The model under review builds one solid part; all positions refer to its coordinate system, in mm. Face numbers are marked on the shaded views. A direction names the side the tool comes from. Round coordinates to 2 decimals unless told otherwise and drop trailing zeros. Order: outer loops, then holes, each group sorted by start corner. A loop starts at its lowest first (then second) coordinate and runs counter-clockwise, first axis right, second up. Notation, with made-up numbers: (-33.75, 67) -> (-14.75, 67) arc R12 ccw to (-14.75, 83) -> close; hole circle Ø3 at (75, 85.5). An arc over 180 degrees is marked (long way). Use a Markdown table: item, result. Add a question column.
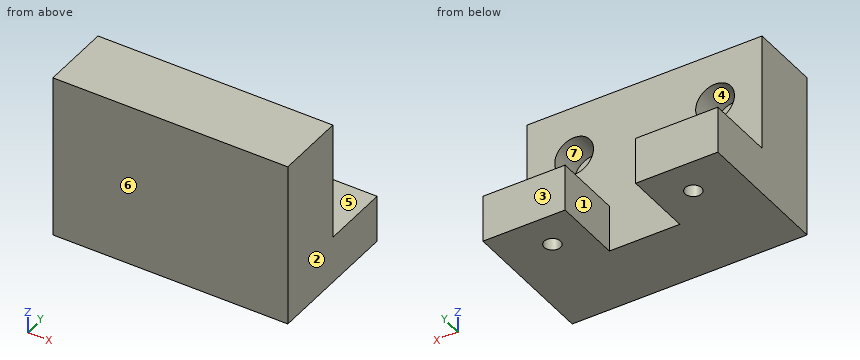
```python
from build123d import *

# Parameters (mm, degrees)
F1_DEPTH = 100
F2_R     = 8.25
F3_DEPTH = 12.954
F4_R     = 3.5
F5_DEPTH = 20
F6_W     = 30
F6_H     = 29.45
F7_DEPTH = 20


with BuildPart() as f1:
    # F0 (on Right) → F1 (new body)
    with BuildSketch(Plane.YZ):
        Polygon((0, 0), (59.45, 0), (59.45, 20), (30, 20), (30, 70), (0, 70), align=None)
    extrude(amount=F1_DEPTH)

    # F2 (on face) → F3 (cut)
    with BuildSketch(Plane(origin=(0, 30, 0), x_dir=(-1, 0, 0), z_dir=(0, 1, 0))):
        with Locations((-80, 48.25)):
            Circle(F2_R)
        with Locations((-20, 48.25)):
            Circle(F2_R)
    extrude(amount=-F3_DEPTH, mode=Mode.SUBTRACT)

    # F4 (on face) → F5 (cut, through all)
    with BuildSketch(Plane.XY.offset(20)):
        with Locations((80, 44.45)):
            Circle(F4_R)
        with Locations((20, 44.45)):
            Circle(F4_R)
    extrude(amount=-F5_DEPTH, mode=Mode.SUBTRACT)

    # F6 (on face) → F7 (cut, through all)
    with BuildSketch(Plane.XY.offset(20)):
        with Locations((50, 44.725)):
            Rectangle(F6_W, F6_H)
    extrude(amount=-F7_DEPTH, mode=Mode.SUBTRACT)


solid = f1.part
```
Q1. For pin 1 (14.5 mm diameter, centred on x = 19, y = 39, fed in from +Z); pin 2 (18 mm diameter, centred on x = 16, z = 47, fed in from +Y); pin 3 (5.5 mm diameter, centred on x = 20, y = 44.45, fed in from -Z), all flat-tipped, find the tip position at first contact; note any pin that passes through.
Q2. Add section A-A, the plane y = 44.45. Give the boundary of the cut face in (x, z), then the cut area to 3 significant figures.
Q3. Draft analysis for pull direction X (two halves, no side actions). For the marked faces 1, 2, 3 and 4, state which applies: released by +X, released by -X, zero draft, split by the parting line, or undercut.
Q4. Add section C-C, the plane y = 32. Give the boundary of the cut face in (x, z), then the cut area to 3 significant figures.
Q5. Add section D-D, the plane z = 48.25. Give the boundary of the cut face in (x, y).
Q6. To check wall thickness, follow line 1 along X through (y, z) = (24, 48); line 2 along Y through (x, z) = (20, 8.75); line 3 along X through (y, z) = (48, 18.5). State the ranges of each line that lie inside material, in increasing order.
Q7. Add section B-B, the plane x = 80. Give the boundary of the cut face in (y, z).
Q8. For the marked faces 5, 6 and 7, list the 3-axis set-ups (+Z, -Z, +X, -X, +Y, -Y) from which the entire face can be reached by the end or side of a thin tool; tool diameter is ignored.
Return value:
| question | item | result |
|---|---|---|
| 1 | pin 1 | z = 20 |
| 1 | pin 2 | y = 30 |
| 1 | pin 3 | through |
| 2 | outline | (0, 0) -> (16.5, 0) -> (16.5, 20) -> (0, 20) -> close; (23.5, 0) -> (35, 0) -> (35, 20) -> (23.5, 20) -> close; (65, 0) -> (76.5, 0) -> (76.5, 20) -> (65, 20) -> close; (83.5, 0) -> (100, 0) -> (100, 20) -> (83.5, 20) -> close |
| 2 | area | 1,120 mm² |
| 3 | face 1 | undercut |
| 3 | face 2 | released by +X |
| 3 | face 3 | zero draft |
| 3 | face 4 | undercut |
| 4 | outline | (0, 0) -> (35, 0) -> (35, 20) -> (0, 20) -> close; (65, 0) -> (100, 0) -> (100, 20) -> (65, 20) -> close |
| 4 | area | 1,400 mm² |
| 5 | outline | (0, 0) -> (100, 0) -> (100, 30) -> (88.25, 30) -> (88.25, 17.05) -> (71.75, 17.05) -> (71.75, 30) -> (28.25, 30) -> (28.25, 17.05) -> (11.75, 17.05) -> (11.75, 30) -> (0, 30) -> close |
| 6 | line 1 | 0 to 11.75, 28.25 to 71.75, 88.25 to 100 |
| 6 | line 2 | 0 to 40.95, 47.95 to 59.45 |
| 6 | line 3 | 0 to 35, 65 to 100 |
| 7 | outline | (0, 0) -> (40.95, 0) -> (40.95, 20) -> (30, 20) -> (30, 40) -> (17.05, 40) -> (17.05, 56.5) -> (30, 56.5) -> (30, 70) -> (0, 70) -> close; (47.95, 0) -> (59.45, 0) -> (59.45, 20) -> (47.95, 20) -> close |
| 8 | face 5 | +Z, +X, -X, +Y |
| 8 | face 6 | +Z, -Z, +X, -X, -Y |
| 8 | face 7 | +Y |
